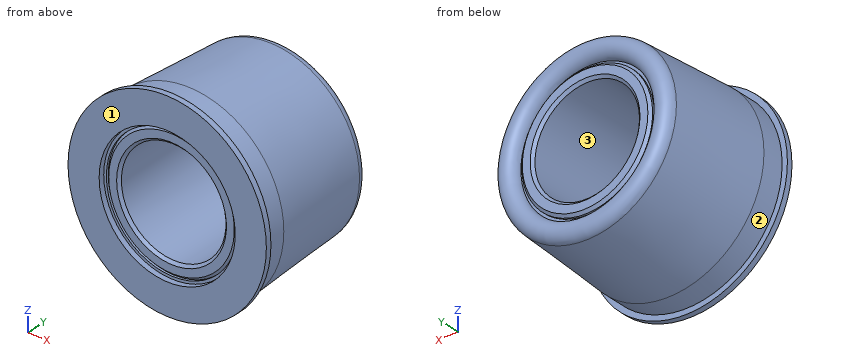
from build123d import *

# Parameters (mm, degrees)
SKETCH3_W     = 1.885
SKETCH3_H     = 18.0848
CHAMFER1_SIZE = 0.37575
SKETCH4_W     = 0.38
SKETCH4_H     = 17.367868501


with BuildPart() as part:
    # Sketch2 → Outer (revolve)
    with BuildSketch(Plane.XY):
        with BuildLine():
            Line((-14.25, -9.8), (-14.25, -9))
            Line((-14.25, -9), (-13.49, -9))
            Line((-13.49, -9), (-13.49, -5.825))
            Line((-13.49, -5.825), (-12.6417422, 8.452803027))
            ThreePointArc((-12.6417422, 8.452803027), (-11.169645536, 9.799369662), (-9.78, 8.367868501))
            Line((-9.78, 8.367868501), (-9.78, -9.8))
            Line((-9.78, -9.8), (-14.25, -9.8))
        make_face()
    revolve(axis=Axis((0, -9.0424, 0), (0, 1, 0)))



with BuildPart() as body_2:
    # Sketch3 → Inner (revolve)
    with BuildSketch(Plane.XY):
        with Locations((-8.4575, 0)):
            Rectangle(SKETCH3_W, SKETCH3_H)
    revolve(axis=Axis((0, -9.0424, 0), (0, 1, 0)))

    # Chamfer1
    chamfer1_edges = [body_2.edges().sort_by_distance(p)[0] for p in [
        (7.515, 9.0424, 0),
        (7.515, -9.0424, 0),
        (9.4, -9.0424, 0),
        (9.4, 9.0424, 0),
    ]]
    chamfer(chamfer1_edges, length=CHAMFER1_SIZE)


with BuildPart() as part_1:
    add(part.part)

    add(body_2.part)  # Combine merges body 2
    # Sketch4 → Combine (revolve)
    with BuildSketch(Plane.XY):
        with Locations((-9.59, -0.316065749)):
            Rectangle(SKETCH4_W, SKETCH4_H)
    revolve(axis=Axis((0, -9.0424, 0), (0, 1, 0)))


solid = part_1.part
Build history of the part. All positions in model axes, mm. Face numbers are marked on the shaded views. Coordinates: 2 decimals unless noted, no trailing zeros. Order: outer loops, then holes, each group sorted by start corner. A loop starts at its lowest first (then second) coordinate and runs counter-clockwise, first axis right, second up. Notation, with made-up numbers: (-12.5, -12.75) - (27.5, -12.75) arc R35 cw to (27.5, 19.25) - close; hole circle Ø4 at (-35, 58.5). An arc over 180 degrees is marked (long way). Put each result on its own line as item: value.
1. Probe line 1 along Z through (x, y) = (0, -9.25); line 2 along Z through (x, y) = (2.25, -7.25); line 3 along X through (y, z) = (-2.5, -1). List the from-to ranges inside material, lowest first. Write a range as [from, to].
Answer sheet:
line 1: z = [-14.25, -9.78], [9.78, 14.25]
line 2: z = [-13.3, -7.17], [7.17, 13.3]
line 3: x = [-13.25, -7.45], [7.45, 13.25]
2. Pull direction X, two halves, no side cores. Call the marked faces 1, 2 and 3: pulls with the +X half, pulls with the -X half, needs draft (parallel to the pull), parting line crosses it, or undercut.
Answer sheet:
face 1: needs draft
face 2: parting line crosses it
face 3: undercut
3. Saw through at A-A (y = -8.25). Write the cut outline in (x, z) (3 decimals).
Answer sheet:
outline: circle Ø26.98 at (0, 0); hole circle Ø15.03 at (0, 0)
4. Drop flat-ended pins along their axis: P1, Ø5, axis at y = -2, z = -0.5, coming from the +X side; P2, Ø15.5, axis at x = -1, z = 3, coming from the +Y side; P3, Ø1.5, axis at x = 7.5, y = 1.5, coming from the +Z side; P4, Ø5.5, axis at x = 3, z = -3, coming from the +Y side. Give the stop position or say it passes through.
Answer sheet:
P1: stops at x = 13.41
P2: stops at y = 9.77
P3: stops at z = 11.18
P4: passes through
5. Saw through at B-B (y = 3). Write the cut outline in (x, z) (3 decimals).
Answer sheet:
outline: circle Ø25.931 at (0, 0); hole circle Ø15.03 at (0, 0)
